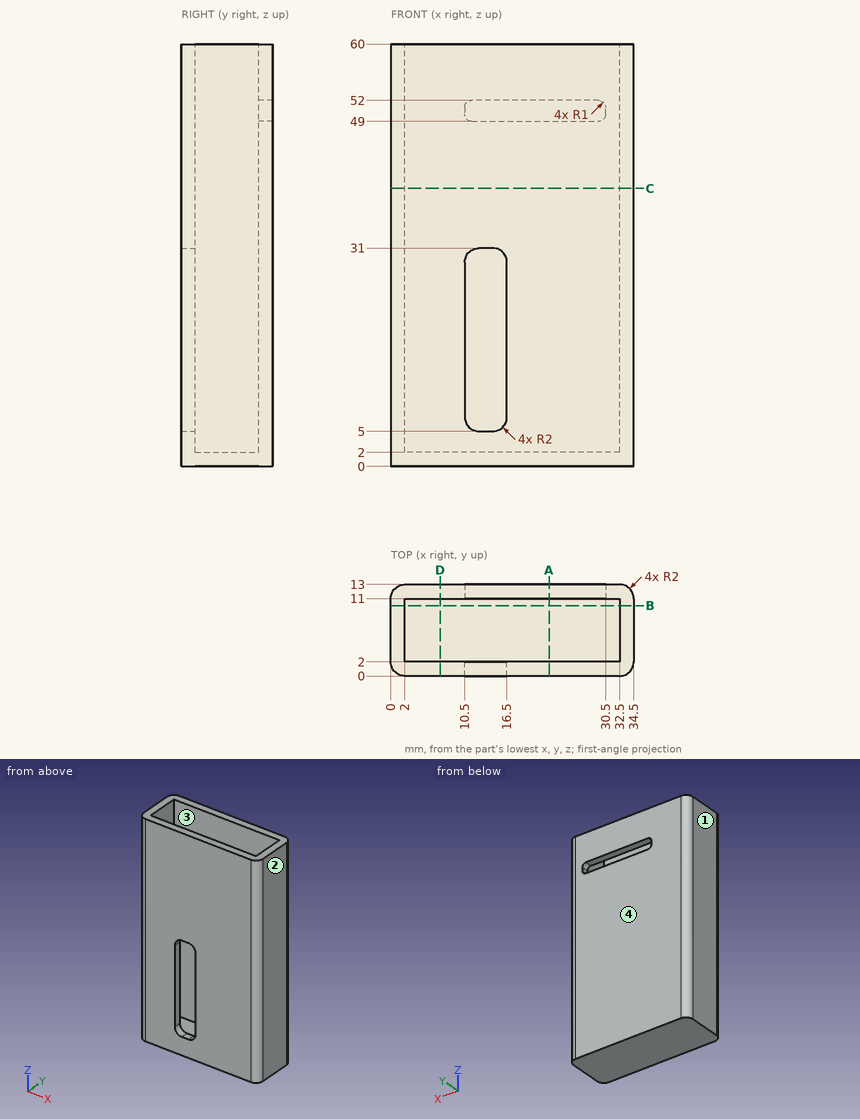
Job drawing, mm, ordinate dimensions from the low corner. One solid piece. Coordinates: 2 decimals unless noted, no trailing zeros. Write each loop counter-clockwise with the first axis right and the second up, starting at its lowest first coordinate (ties: lowest second). Pieces come first, ordered by that corner, then holes. Notation, with made-up numbers: (20.5, 73.5) -> (74.5, 73.5) arc R23 cw to (74.5, 96.5) -> close; hole circle Ø6 at (45.5, -18). An arc over 180 degrees is marked (long way). Use CSV: the item, a comma, the result in double quotes. Start each with the question number.
Item 1: Wall check: probe 1 along X at (y, z) = (5.25, 20); probe 2 along Y at (x, z) = (27.5, 8.5); probe 3 along Y at (x, z) = (15, 20). Give the ranges that are in metal, low to high.
Item 2: Drop flat-ended pins along their axis: P1, Ø1.6, axis at y = 1, z = 23.5, coming from the +X side; P2, Ø0.5, axis at y = 11.5, z = 50.5, coming from the -X side; P3, Ø7, axis at x = 9.5, y = 7, coming from the +Z side. Give the stop position or say it passes through.
Item 3: Two-plate mould, pull along X, no slides. Class the marked faces 1, 2, 3 and 4: +X half, -X half, draft (parallel to the pull), parting line (faces both ways), or undercut.
Item 4: Band-saw the part on B-B, the plane y = 10. Write the cut outline in (x, z), plus the area to 3 significant figures.
Item 5: Band-saw the part on C-C, the plane z = 39.5. Write the cut outline in (x, y).
Item 6: Band-saw the part on D-D, the plane x = 7. Write the cut outline in (y, z), plus the area to 3 significant figures.
Item 7: Band-saw the part on A-A, the plane x = 22.5. Write the cut outline in (y, z), plus the area to 3 significant figures.
Response values:
1,probe 1,"x = 0 to 2, 32.5 to 34.5"
1,probe 2,"y = 0 to 2, 11 to 13"
1,probe 3,"y = 11 to 13"
2,P1,"stops at x = 34.49"
2,P2,"stops at x = 0.02"
2,P3,"stops at z = 2"
3,face 1,"-X half"
3,face 2,"+X half"
3,face 3,"undercut"
3,face 4,"draft"
4,outline,"(0, 0) -> (34.5, 0) -> (34.5, 60) -> (32.5, 60) -> (32.5, 2) -> (2, 2) -> (2, 60) -> (0, 60) -> close"
4,area,"301 mm2"
5,outline,"(0, 2) arc R2 ccw to (2, 0) -> (32.5, 0) arc R2 ccw to (34.5, 2) -> (34.5, 11) arc R2 ccw to (32.5, 13) -> (2, 13) arc R2 ccw to (0, 11) -> close; hole (2, 2) -> (32.5, 2) -> (32.5, 11) -> (2, 11) -> close"
6,outline,"(0, 0) -> (13, 0) -> (13, 60) -> (11, 60) -> (11, 2) -> (2, 2) -> (2, 60) -> (0, 60) -> close"
6,area,"258 mm2"
7,outline,"(0, 0) -> (13, 0) -> (13, 49) -> (11, 49) -> (11, 2) -> (2, 2) -> (2, 60) -> (0, 60) -> close; (11, 52) -> (13, 52) -> (13, 60) -> (11, 60) -> close"
7,area,"252 mm2"
